Autodesk Inventor part; units mm, degrees
ref_plane "YZ Plane" through (0, 0, 0) normal (1, 0, 0) x (0, 1, 0)
ref_plane "XZ Plane" through (0, 0, 0) normal (0, 1, 0) x (-1, 0, 0)
ref_plane "XY Plane" through (0, 0, 0) normal (0, 0, 1) x (1, 0, 0)
sketch "スケッチ1" plane through (0, 0, 0) normal (0, 0, 1) x (1, 0, 0)
  line L0 (0, 0) -> (352, 0)
  line L1 (352, 0) -> (352, 5)
  line L2 (352, 5) -> (0, 5)
  line L3 (0, 5) -> (0, 0)
  line L4 (0, 0) -> (6, 0)
  line L5 (0, 1) -> (0, 0)
  dimension "d0" = 352
  dimension "d1" = 5
extrude "押し出し1" add sketch "スケッチ1" along normal blind 20
sketch "スケッチ3" plane through (0, 0, 0) normal (-1, 0, 0) x (0, 0, 1)
  line L0 (0, 5) -> (0, 0)
  line L1 (0, 0) -> (20, 0)
  line L2 (20, 5) -> (20, 0)
  line L3 (0, 5) -> (20, 5)
  circle A0 centre (4, 2) radius 1.2
  circle A1 centre (16, 3) radius 1.2
  dimension "d14" = 2.4
  dimension "d15" = 2.4
  dimension "d16" = 3
  dimension "d17" = 4
  dimension "d18" = 4
  dimension "d19" = 3
extrude "押し出し3" cut sketch "スケッチ3" against normal blind 6 contours A0 | A1
sketch "スケッチ4" plane through (0, 0, 0) normal (0, -1, 0) x (1, 0, 0)
  line L0 (0, 0) -> (352, 0)
  line L1 (352, 0) -> (352, 20)
  line L2 (0, 20) -> (352, 20)
  line L3 (0, 0) -> (0, 20)
  line L4 (2, 2) -> (350, 2)
  line L5 (350, 2) -> (350, 18)
  line L6 (350, 18) -> (2, 18)
  line L7 (2, 18) -> (2, 2)
  dimension "d22" = 2
  dimension "d23" = 2
  dimension "d24" = 2
  dimension "d25" = 2
extrude "押し出し4" cut sketch "スケッチ4" against normal blind 3 contours L7 L6 L5 L4
sketch "スケッチ5" plane through (0, 5, 0) normal (0, 1, 0) x (1, 0, 0)
  circle A0 centre (322, -10) radius 8
extrude "押し出し5" cut sketch "スケッチ5" against normal through all
sketch "スケッチ6" plane through (0, 5, 0) normal (0, 1, 0) x (1, 0, 0)
  circle A0 centre (340, -10) radius 3
extrude "押し出し6" cut sketch "スケッチ6" against normal through all
sketch "スケッチ7" plane through (0, 5, 0) normal (0, 1, 0) x (1, 0, 0)
  circle A0 centre (309.5, -10) radius 2.5
  circle A1 centre (288.5, -10) radius 2
  circle A2 centre (276.5, -10) radius 2.5
extrude "押し出し7" cut sketch "スケッチ7" against normal through all
sketch "スケッチ8" plane through (0, 0, 20) normal (0, 0, 1) x (1, 0, 0)
  line L0 (352, 5) -> (0, 5)
  line L1 (0, 5) -> (0, 0)
  line L2 (0, 0) -> (352, 0)
  line L3 (350, 0) -> (2, 0)
  line L4 (0, 5) -> (12, 5)
  line L5 (12, 5) -> (12, 0)
  line L6 (12, 0) -> (0, 0)
  line L7 (0, 0) -> (0, 5)
  dimension "d34" = 12
extrude "押し出し8" cut sketch "スケッチ8" against normal through all
sketch "スケッチ9" plane through (0, 3, 0) normal (0, -1, 0) x (1, 0, 0)
  line L0 (12, 0) -> (12, 20)
  line L1 (12, 10) -> (22, 10)
  circle A0 centre (22, 10) radius 3
  point P0 (0, 0)
  dimension "d37" = 10
  dimension "d38" = 6
extrude "押し出し9" cut sketch "スケッチ9" against normal through all
fillet "フィレット1" radius 10 2 edges at (12, 2.5, 20) (12, 2.5, 0)
properties part number "arm1_L"
Read the model definition and answer for the solid it produces. Units are mm, in the model's axes. A direction names the side the tool comes from. Coordinates: 2 decimals unless noted, no trailing zeros. Write each loop counter-clockwise with the first axis right and the second up, starting at its lowest first coordinate (ties: lowest second). Pieces come first, ordered by that corner, then holes. Notation, with made-up numbers: M 10,86 L 60,86 A17 cw 60,114 Z; hole C -18.5,42 d11. An arc over 180 degrees is marked long. Use a Markdown table: item, result.
Q1. Determine the mould class of faces 1 (the face through (16, 4, 2)), 2 (the face through (184, 5, 10)), 3 (the face through (336, 3, 10)) for opening direction Z: released by +Z, released by -Z, zero draft, split by the parting line, or undercut.
Answer block:
| item | result |
|---|---|
| face 1 | released by -Z |
| face 2 | zero draft |
| face 3 | undercut |
Q2. This flat-tipped pin is pushed along its axis until it touches: pin 1 Ø1 at (y, z) = (1.5, 5.5) entering from -X. Where does it stop, or does it pass through?
Answer block:
| item | result |
|---|---|
| pin 1 | stops at x = 350 |
Q3. Which of the six approach directions +Z, -Z, +X, -X, +Y, -Y give full straight-line access (tool end or side, diameter ignored) to faces 4 (the face through (165, 3, 10)), 5 (the face through (16.35, 3.02, 18.25))?
Answer block:
| item | result |
|---|---|
| face 4 | -X, -Y |
| face 5 | +Z, -X, +Y, -Y |
Q4. Straight lines are drawn through the part: L1, parallel to Z at x = 319.5, y = 0.65; L2, parallel to Z at x = 309.5, y = 4.6; L3, parallel to X at y = 2, z = 16.5. For each, find the intervals that lie inside material, in ascending order. Write a range as [from, to].
Answer block:
| item | result |
|---|---|
| L1 | z = [0, 2], [18, 20] |
| L2 | z = [0, 7.5], [12.5, 20] |
| L3 | x = [350, 352] |
Q5. The part is cut by section A-A, the plane y = 4. Give the number of separate pieces and of enclosed holes in the cut face, then the cut area to 3 significant figures.
Answer block:
| item | result |
|---|---|
| separate pieces | 1 |
| enclosed holes | 6 |
| area | 6,450 mm2 |
Q6. The part is cut by section B-B, the plane x = 38. Write down the section's boundary in (y, z).
Answer block:
| item | result |
|---|---|
| outline | M 0,0 L 5,0 L 5,20 L 0,20 L 0,18 L 3,18 L 3,2 L 0,2 Z |
